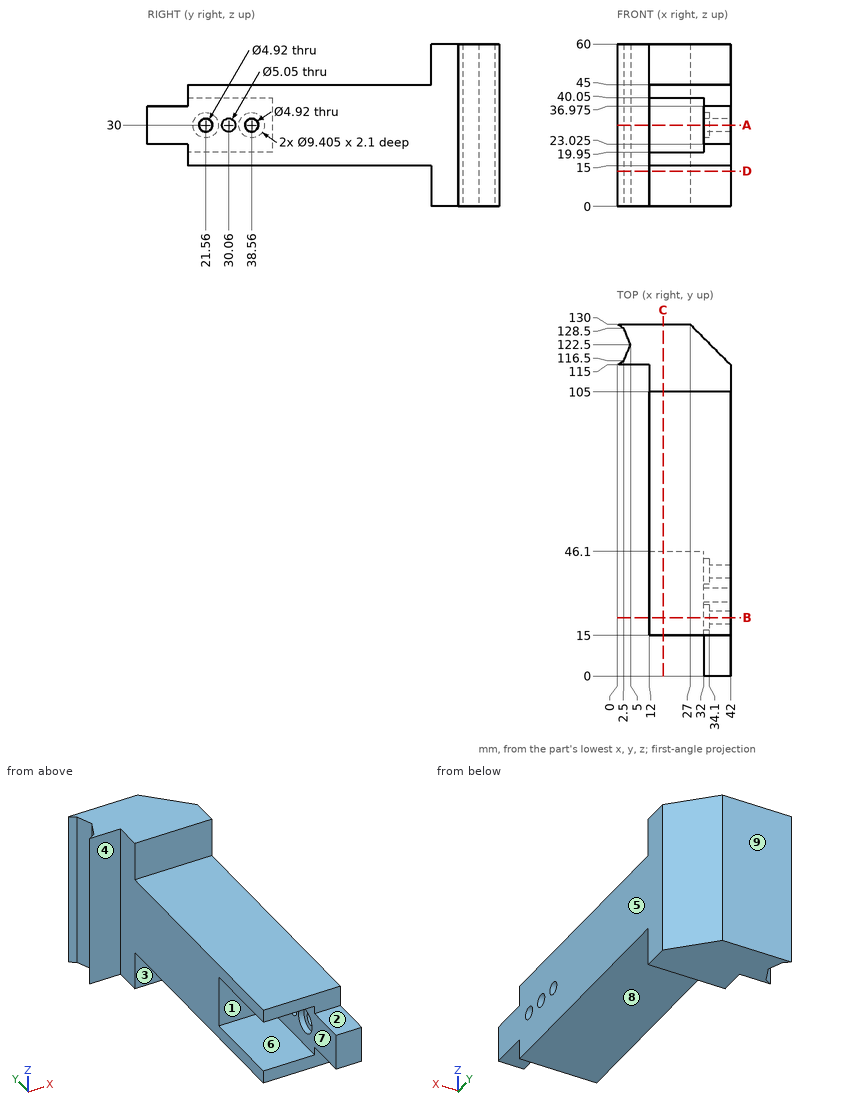
Input: dimensioned drawing with shaded views. Units: mm. Origin: part minimum x, y, z. A direction names the side the tool comes from. Give positions to 0.01 mm unless a question says otherwise; leave off trailing zeros. Write each loop counter-clockwise with the first axis right and the second up, starting at its lowest first coordinate (ties: lowest second). Pieces come first, ordered by that corner, then holes. Notation, with made-up numbers: M 39,-36 L 76,-36 A22 cw 76,-23 Z; hole C 26.25,84.5 d10. An arc over 180 degrees is marked long. Return JSON: item names as keys, results as strings. Group by question number.
1) Cut plane A-A, the plane z = 30. Give the number of separate pieces and of enclosed holes in the cut face, plus the area to 3 significant figures.
2) Cut plane D-D, the plane z = 13. Output: boundary loops of the cut face in (x, y), plus the area to 3 significant figures.
3) Pin query (flat end, axial travel): P1, Ø10, axis at x = 20, z = 28, coming from the -Y side; P2, Ø9.5, axis at x = 3, z = 20.5, coming from the -Y side; P3, Ø2, axis at x = 13, y = 97.5, coming from the +Z side. Return the tip coordinate at first contact, or that it passes through.
4) Pull-direction query (Z, two-part tool) for the marked faces 6, 7, 8 and 9; classes: pulls with the +Z half, pulls with the -Z half, needs draft (parallel to the pull), parting line crosses it, or undercut.
5) Cut plane C-C, the plane x = 17. Output: boundary loops of the cut face in (y, z), plus the area to 3 significant figures.
6) Cut plane B-B, the plane y = 21.56. Output: boundary loops of the cut face in (x, z).
7) Set-up query: the marked faces 1, 2, 3, 4 and 5. Return all of +Z, -Z, +X, -X, +Y, -Y with unobstructed straight access to the full face (end or side cutting, diameter ignored); none if empty.
8) Material intervals for line 1 along Y through (x, z) = (40.5, 30) (3 decimals); line 2 along Y through (x, z) = (39.5, 30) (3 decimals); line 3 along Z through (x, y) = (18, 18), sorted ascending. Write a range as [from, to].
Recorded:
{
 "1": {"separate pieces": "4", "enclosed holes": "0", "area": "2,830 mm²"},
 "2": {"outline": "M 0,115 L 12,115 L 12,105 L 42,105 L 42,115 L 27,130 L 0,130 L 2.5,128.5 L 5,122.5 L 2.5,116.5 Z", "area": "769 mm²"},
 "3": {"P1": "stops at y = 46.1", "P2": "stops at y = 115", "P3": "stops at z = 45"},
 "4": {"face 6": "undercut", "face 7": "undercut", "face 8": "pulls with the -Z half", "face 9": "needs draft"},
 "5": {"outline": "M 15,15 L 105,15 L 105,0 L 130,0 L 130,60 L 105,60 L 105,45 L 15,45 L 15,40.05 L 46.1,40.05 L 46.1,19.95 L 15,19.95 Z", "area": "3,570 mm²"},
 "6": {"outline": "M 12,15 L 42,15 L 42,27.54 L 34.1,27.54 L 34.1,25.3 L 32,25.3 L 32,19.95 L 12,19.95 Z; M 12,40.05 L 32,40.05 L 32,34.7 L 34.1,34.7 L 34.1,32.46 L 42,32.46 L 42,45 L 12,45 Z"},
 "7": {"face 1": "-X, -Y", "face 2": "+Z, +X, -X, -Y", "face 3": "-Z, +X, -X, -Y", "face 4": "+Z, -Z, -X, -Y", "face 5": "+Z, -Z, +X, +Y, -Y"},
 "8": {"line 1": "y = [0, 19.1], [24.02, 27.535], [32.585, 36.1], [41.02, 116.5]", "line 2": "y = [0, 19.1], [24.02, 27.535], [32.585, 36.1], [41.02, 117.5]", "line 3": "z = [15, 19.95], [40.05, 45]"}
}
